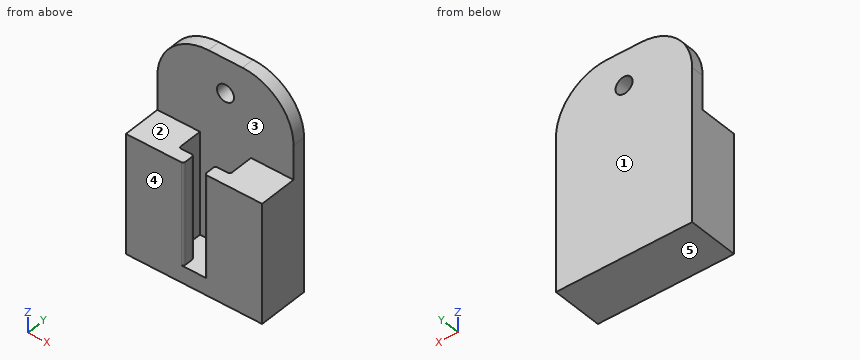
from build123d import *

# Parameters (mm, degrees)
F0_W      = 25.4
F0_H      = 38.1
F1_DEPTH  = 9.525
F2_W      = 3.96875
F2_H      = 2.38125
F3_DEPTH  = 22.225
F4_W      = 25.4
F4_H      = 15.875
F5_DEPTH  = 7.14375
F6_R      = 9.525
F7_R      = 0.396875
F8_W      = 25.4
F8_H      = 9.525
F9_DEPTH  = 3.175
F10_R     = 1.5875
F11_DEPTH = 2.38225


with BuildPart() as f1:
    # F0 (on Front) → F1 (new body)
    with BuildSketch(Plane.XZ):
        with Locations((0, 19.05)):
            Rectangle(F0_W, F0_H)
    extrude(amount=F1_DEPTH)

    # F2 (on Top) → F3 (cut)
    with BuildSketch(Plane.XY):
        Polygon((4.7625, -2.38125), (-4.7625, -2.38125), (-4.7625, -7.14375), (-1.984375, -7.14375), (1.984375, -7.14375), (4.7625, -7.14375), align=None)
        with Locations((0, -8.334375)):
            Rectangle(F2_W, F2_H)
    extrude(amount=F3_DEPTH, mode=Mode.SUBTRACT)

    # F4 (on face) → F5 (cut)
    with BuildSketch(Plane.XZ.offset(9.525)):
        with Locations((0, 30.1625)):
            Rectangle(F4_W, F4_H)
    extrude(amount=-F5_DEPTH, mode=Mode.SUBTRACT)

    # F6
    f6_edges = [f1.edges().sort_by_distance(p)[0] for p in [
        (12.7, -1.190625, 38.1),
        (-12.7, -1.190625, 38.1),
    ]]
    fillet(f6_edges, radius=F6_R)

    # F7
    f7_edges = [f1.edges().sort_by_distance(p)[0] for p in [
        (-4.7625, -7.14375, 11.1125),
        (4.7625, -7.14375, 11.1125),
        (1.984375, -7.14375, 11.1125),
        (1.984375, -9.525, 11.1125),
        (-1.984375, -7.14375, 11.1125),
        (-1.984375, -9.525, 11.1125),
    ]]
    fillet(f7_edges, radius=F7_R)

    # F8 (on face) → F9 (join)
    with BuildSketch(Plane(origin=(0, 0, 0), x_dir=(1, 0, 0), z_dir=(0, 0, -1))):
        with Locations((0, 4.7625)):
            Rectangle(F8_W, F8_H)
    extrude(amount=-F9_DEPTH)

    # F10 (on face) → F11 (cut, through all)
    with BuildSketch(Plane.XZ.offset(2.38125)):
        with Locations((0, 31.75)):
            Circle(F10_R)
    extrude(amount=-F11_DEPTH, mode=Mode.SUBTRACT)


solid = f1.part
Can you work these out from the model? Positions are in its coordinate system, mm. Face numbers are marked on the shaded views. A direction names the side the tool comes from. Give positions to 0.01 mm unless a question says otherwise; leave off trailing zeros. Order: outer loops, then holes, each group sorted by start corner. A loop starts at its lowest first (then second) coordinate and runs counter-clockwise, first axis right, second up. Notation, with made-up numbers: (81, 41.5) - (97, 41.5) arc R11 cw to (97, 62.5) - close; hole circle Ø9 at (84, 72.5). An arc over 180 degrees is marked (long way). Write each question's results on one line, items separated by ' | '.
1) Suppose I cut it at C-C, the plane y = -4.5. Write out the boundary of the cut face in (x, z) (1 decimal).
Final values:
outline: (-12.7, 0) - (12.7, 0) - (12.7, 22.2) - (4.8, 22.2) - (4.8, 3.2) - (-4.8, 3.2) - (-4.8, 22.2) - (-12.7, 22.2) - close
2) Please list where these lines run through material, in increasing order: line 1 along X through (y, z) = (-6.5, 21.5); line 2 along Z through (x, y) = (0, -1.75); line 3 along Y through (x, z) = (-3.5, 6.5) (3 decimals). Write a range as [from, to].
Final values:
line 1: x = [-12.7, -4.76], [4.76, 12.7] | line 2: z = [0, 30.16], [33.34, 38.1] | line 3: y = [-9.525, -7.144], [-2.381, 0]
3) Suppose I cut it at D-D, the plane z = 7. Write out the boundary of the cut face in (x, y) (1 decimal), then the cut area to 3 significant figures.
Final values:
outline: (-12.7, -9.5) - (-2.4, -9.5) arc R0.4 ccw to (-2, -9.1) - (-2, -7.5) arc R0.4 ccw to (-2.4, -7.1) - (-4.4, -7.1) arc R0.4 cw to (-4.8, -6.7) - (-4.8, -2.4) - (4.8, -2.4) - (4.8, -6.7) arc R0.4 cw to (4.4, -7.1) - (2.4, -7.1) arc R0.4 ccw to (2, -7.5) - (2, -9.1) arc R0.4 ccw to (2.4, -9.5) - (12.7, -9.5) - (12.7, 0) - (-12.7, 0) - close | area: 187 mm^2
4) I'm going to push flat-ended pins straight in: pin 1 Ø1.6 at (x, z) = (-4, 15.5) entering from +Y; pin 2 Ø2 at (x, y) = (3.5, -8) entering from +Z (3 decimals); pin 3 Ø5 at (x, z) = (0, 31.75) entering from -Y; pin 4 Ø3 at (x, y) = (6, -1.5) entering from +Z. Where does each tip first touch, or does it pass through?
Final values:
pin 1: stops at y = 0 | pin 2: stops at z = 22.225 | pin 3: stops at y = -2.38 | pin 4: stops at z = 38.01
5) If we mould it in two halves opening along Y, with no side actions, what happens to the marked faces 3, 4 and 5? For each: pulls with the +Y half, pulls with the -Y half, needs draft (parallel to the pull), parting line crosses it, or undercut.
Final values:
face 3: undercut | face 4: pulls with the -Y half | face 5: needs draft
6) Suppose I cut it at A-A, the plane x = 0. Write out the boundary of the cut face in (y, z) (1 decimal), then the cut area to 3 significant figures.
Final values:
outline: (-9.5, 0) - (0, 0) - (0, 30.2) - (-2.4, 30.2) - (-2.4, 3.2) - (-9.5, 3.2) - close; (-2.4, 33.3) - (0, 33.3) - (0, 38.1) - (-2.4, 38.1) - close | area: 106 mm^2
7) Suppose I cut it at B-B, the plane z = 31.75. Write out the boundary of the cut face in (x, y), then the cut area to 3 significant figures.
Final values:
outline: (-12.16, -2.38) - (-1.59, -2.38) - (-1.59, 0) - (-12.16, 0) - close; (1.59, -2.38) - (12.16, -2.38) - (12.16, 0) - (1.59, 0) - close | area: 50.3 mm^2
8) On a 3-axis mill with a long thin cutter (end or side, diameter ignored), from which of +Z, -Z, +X, -X, +Y, -Y can I reach the whole of each face in a straight line? I mean the marked faces 1 and 2. Say none if no direction works.
Final values:
face 1: +Z, -Z, +X, -X, +Y | face 2: +Z, +X, -X, -Y
